Solid Edge part; units mm, degrees
sketch "Sketch1" plane through (0, 0, 0) normal (1, 0, 0) x (0, 1, 0)
  circle A0 centre (0, 0) radius 2
extrude "Protrusion1" add sketch "Sketch1" along normal mid plane 46
chamfer "Chamfer_1" distance 0.5 angle 45 2 edges at (23, -2, 0) (-23, -2, 0)
sketch "Sketch2" plane through (0, 0, 0) normal (0, -1, 0) x (1, 0, 0)
  line L0 (20.5, 2) -> (20.5, 1.5)
  line L1 (20.5, 1.5) -> (20, 1.5)
  line L2 (20, 1.5) -> (20, 2)
  line L3 (20, 2) -> (20.5, 2)
revolve "RevolvedCutout1" cut sketch "Sketch2" angle 360 about axis through (23, 0, 0) along (-1, 0, 0)
mirror "Mirror1" about plane through (0, 0, 0) normal (1, 0, 0) of "RevolvedCutout1"
properties material "PVC"
Geometry: final body of the model. Coordinates: model frame, mm. A direction names the side the tool comes from. Round coordinates to 2 decimals unless told otherwise and drop trailing zeros. Order: outer loops, then holes, each group sorted by start corner. A loop starts at its lowest first (then second) coordinate and runs counter-clockwise, first axis right, second up. Notation, with made-up numbers: (5.5, 22) -> (48.5, 22) arc R18 ccw to (48.5, 40) -> close; hole circle Ø9 at (81, 71.25). An arc over 180 degrees is marked (long way). Use one line per item in the form item = value.
(1) Ray query, probe 1 along X at (y, z) = (1.8, 0.7); probe 2 along X at (y, z) = (1.8, 0.1); probe 3 along Y at (x, z) = (5.5, 0.2). Return the intervals inside material, ascending. Write a range as [from, to].
Results list:
probe_1 = [-22.57, -20.5], [-20, 20], [20.5, 22.57]
probe_2 = [-22.7, -20.5], [-20, 20], [20.5, 22.7]
probe_3 = [-1.99, 1.99]
(2) Access query for faces 4 (the face through (-20.25, -0.07, -1.5)), 5 (the face through (-21, 0, -2)). Directions: +Z, -Z, +X, -X, +Y, -Y. A direction counts if a zero-diameter tool reaches every point of the face in a straight line with its end or side. Return the directions, or none.
Results list:
face_4 = none
face_5 = +X, -X
(3) Draft query along X for faces 1 (the face through (23, 0, 0)), 2 (the face through (0, 0, 2)), 3 (the face through (20.25, 0.07, -1.5)). Return one class per face: pulls with the +X half, pulls with the -X half, needs draft (parallel to the pull), parting line crosses it, or undercut.
Results list:
face_1 = pulls with the +X half
face_2 = needs draft
face_3 = undercut
(4) Section A-A on x = 19. Return loops of the section in (y, z).
Results list:
outline = circle Ø4 at (0, 0)
